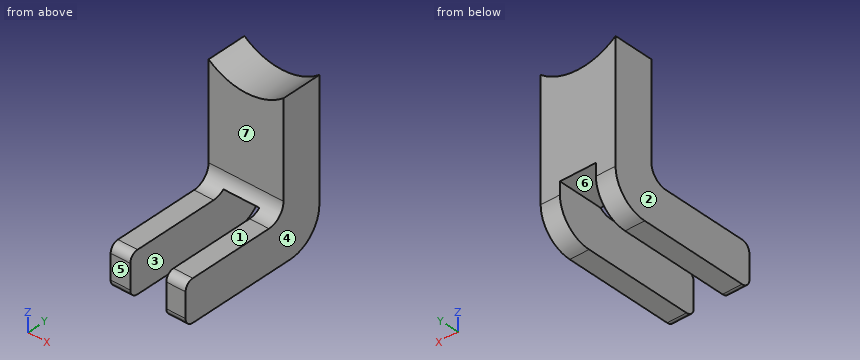
from build123d import *

# Parameters (mm, degrees)
EXTRUDE_START         = -3
EXTRUDE_1_DEPTH       = 46
SKETCH_2_W            = 22
SKETCH_2_H            = 41.003909118
CUT_EXTRUDE_2_DEPTH   = 115
SKETCH_4_W            = 74
SKETCH_4_H            = 24.59688775
EXTRUDE_3_DEPTH       = 55
CUT_EXTRUDE_2_2_DEPTH = 50
FILLET_2_R            = 4
SKETCH_7_R            = 3
CUT_EXTRUDE_3_DEPTH   = 90
FILLET_3_R            = 10
SKETCH_9_W            = 165.264464741
SKETCH_9_H            = 119.978910546
CUT_EXTRUDE_5_DEPTH   = 14.2
SKETCH_10_W           = 169.580693543
SKETCH_10_H           = 115.14513644
CUT_EXTRUDE_6_DEPTH   = 14


with BuildPart() as part:
    # Эскиз1 → Вытянуть1 (new body)
    with BuildSketch(Plane(origin=(0, 0, 0), x_dir=(0, 0, -1), z_dir=(1, 0, 0)).offset(EXTRUDE_START)):
        with BuildLine():
            Line((3.683652722, 0), (3.683652722, -24.59688775))
            Line((3.683652722, -24.59688775), (49.132150834, -24.59688775))
            ThreePointArc((49.132150834, -24.59688775), (56.203218646, -27.525819938), (59.132150834, -34.59688775))
            Line((59.132150834, -34.59688775), (59.132150834, -86.83159597))
            ThreePointArc((59.132150834, -86.83159597), (60.596616928, -90.367129876), (64.132150834, -91.83159597))
            Line((64.132150834, -91.83159597), (79.132150834, -91.83159597))
            ThreePointArc((79.132150834, -91.83159597), (82.66768474, -90.367129876), (84.132150834, -86.83159597))
            Line((84.132150834, -86.83159597), (84.132150834, -20))
            ThreePointArc((84.132150834, -20), (78.274286458, -5.857864376), (64.132150834, 0))
            Line((64.132150834, 0), (3.683652722, 0))
        make_face()
    extrude(amount=EXTRUDE_1_DEPTH)

    # Эскиз2 → Cut-Extrude 2 (cut, symmetric)
    with BuildSketch(Plane(origin=(0, 0, 0), x_dir=(1, 0, 0), z_dir=(0, 1, 0))):
        with Locations((20, 77.079487522)):
            Rectangle(SKETCH_2_W, SKETCH_2_H)
    extrude(amount=CUT_EXTRUDE_2_DEPTH, both=True, mode=Mode.SUBTRACT)

    # Эскиз4 → Вытянуть3 (add)
    with BuildSketch(Plane.XY.offset(-3.683652722)):
        with Locations((20.00338787, -12.298443875)):
            Rectangle(SKETCH_4_W, SKETCH_4_H)
    extrude(amount=EXTRUDE_3_DEPTH)

    # Эскиз6 → Cut-Extrude 2 2 (cut, symmetric)
    with BuildSketch(Plane(origin=(0, 0, 0), x_dir=(1, 0, 0), z_dir=(0, 1, 0))):
        with BuildLine():
            Line((47.00338787, -53.713591308), (47.00338787, -12.467045061))
            ThreePointArc((47.00338787, -12.467045061), (20.003387867, -0.765266351), (-6.99661213, -12.467045078))
            Line((-6.99661213, -12.467045078), (-6.99661213, -53.713591308))
            Line((-6.99661213, -53.713591308), (47.00338787, -53.713591308))
        make_face()
    extrude(amount=CUT_EXTRUDE_2_2_DEPTH, both=True, mode=Mode.SUBTRACT)

    # Скругление2
    fillet_2_edges = [part.edges().sort_by_distance(p)[0] for p in [
        (57.00338787, -12.298443875, -3.683652722),
        (-16.99661213, -12.298443875, -3.683652722),
    ]]
    fillet(fillet_2_edges, radius=FILLET_2_R)

    # Эскиз7 → Вырез-Вытянуть3 (cut, symmetric)
    with BuildSketch(Plane(origin=(57.00338787, 0, 0), x_dir=(0, 0, -1), z_dir=(1, 0, 0))):
        with Locations((-35.623538585, -11.460561108)):
            Circle(SKETCH_7_R)
    extrude(amount=CUT_EXTRUDE_3_DEPTH, both=True, mode=Mode.SUBTRACT)

    # Скругление3
    fillet_3_edges = [part.edges().sort_by_distance(p)[0] for p in [
        (-3, -12.298443875, -3.683652722),
        (43, -12.298443875, -3.683652722),
    ]]
    fillet(fillet_3_edges, radius=FILLET_3_R)

    # Эскиз9 → Вытянуть5 (cut)
    with BuildSketch(Plane(origin=(57.00338787, 0, 0), x_dir=(0, 0, -1), z_dir=(1, 0, 0))):
        with Locations((28.438864211, -53.728415023)):
            Rectangle(SKETCH_9_W, SKETCH_9_H)
    extrude(amount=-CUT_EXTRUDE_5_DEPTH, mode=Mode.SUBTRACT)

    # Эскиз10 → Вытянуть6 (cut)
    with BuildSketch(Plane.ZY.offset(16.99661213)):
        with Locations((-24.768184397, -40.528258671)):
            Rectangle(SKETCH_10_W, SKETCH_10_H)
    extrude(amount=-CUT_EXTRUDE_6_DEPTH, mode=Mode.SUBTRACT)


solid = part.part
The listing builds one solid part. Answer for the finished solid, in the listing's coordinates (mm). Face numbers are marked on the shaded views. A direction names the side the tool comes from. Give positions to 0.01 mm unless a question says otherwise; leave off trailing zeros. Write each loop counter-clockwise with the first axis right and the second up, starting at its lowest first coordinate (ties: lowest second). Pieces come first, ordered by that corner, then holes.
1) Section D-D (y = -15.5) is taken. Write down the section's boundary in (x, z).
2) A tool of negligible diameter and unlimited length cuts with its end or side. For the marked faces 5, 6 and 7, from which of +Z, -Z, +X, -X, +Y, -Y can it reach the whole face along a straight path? Write none if from no direction.
3) Section B-B (z = -75) is taken. Write down the section's boundary in (x, y).
4) For a pull along X with two mould halves and no side action, classify the marked faces 1, 2, 3 and 4 as pulls with the +X half, pulls with the -X half, needs draft (parallel to the pull), parting line crosses it, or undercut.
5) Given P1, Ø13, axis at x = 2, y = -71.5, coming from the +Z side; P2, Ø2, axis at x = 18, z = -19, coming from the +Y side, each flat-ended and moving along its own axis, determine where each tip first touches the part or whether it passes through.
6) Section C-C (x = 40) is taken. Write down the section's boundary in (y, z).
7) Find the intervals of material crossed by L1, parallel to X at y = -17, z = -77.5; L2, parallel to Y at x = 2.5, z = -33.5; L3, parallel to Z at x = 6.5, y = -54, in increasing order.
8) Section A-A (y = -58.5) is taken. Write down the section's boundary in (x, z).
Response:
1. outline: (-3, -83.62) - (9, -83.62) - (9, -56.58) - (31, -56.58) - (31, -83.62) - (42.8, -83.62) - (42.8, 8.62) arc R37 cw to (-3, 8.78) - close
2. face 5: +Z, -Z, +X, -X, -Y
2. face 6: -Z, +Y, -Y
2. face 7: +Z, +X, -X, -Y
3. outline: (-3, -91.83) - (9, -91.83) - (9, -3.21) - (-3, -3.21) - close; (31, -91.83) - (42.8, -91.83) - (42.8, -3.21) - (31, -3.21) - close
4. face 1: needs draft
4. face 2: pulls with the -X half
4. face 3: undercut
4. face 4: pulls with the +X half
5. P1: stops at z = -59.13
5. P2: stops at y = 0
6. outline: (-91.83, -79.13) arc R5 ccw to (-86.83, -84.13) - (-20, -84.13) arc R20 ccw to (0, -64.13) - (0, 6.63) - (-24.6, 6.63) - (-24.6, -49.13) arc R10 cw to (-34.6, -59.13) - (-86.83, -59.13) arc R5 ccw to (-91.83, -64.13) - close
7. L1: x = -3 to 9, 31 to 42.8
7. L2: y = -24.6 to 0
7. L3: z = -84.13 to -59.13
8. outline: (-3, -84.13) - (9, -84.13) - (9, -59.13) - (-3, -59.13) - close; (31, -84.13) - (42.8, -84.13) - (42.8, -59.13) - (31, -59.13) - close
